Autodesk Inventor part; units mm, degrees
ref_plane "YZ Plane" through (0, 0, 0) normal (1, 0, 0) x (0, 1, 0)
ref_plane "XZ Plane" through (0, 0, 0) normal (0, 1, 0) x (-1, 0, 0)
ref_plane "XY Plane" through (0, 0, 0) normal (0, 0, 1) x (1, 0, 0)
sketch "Sketch1" plane through (0, 0, 0) normal (0, 0, 1) x (1, 0, 0)
  arc A0 (4.0641, 0.1774) -> (4.0641, -0.1774) centre (0, 0) ccw
  arc A1 (5.6501, 0.2467) -> (5.6501, -0.2467) centre (0, 0) ccw
  line L0 (4.0641, -0.1774) -> (5.6501, -0.2467)
  line L1 (4.0641, 0.1774) -> (5.6501, 0.2467)
  dimension "d0" = 8.1359
  dimension "d13" = 5
  dimension "d26" = 1.5875
extrude "Extrusion3" add sketch "Sketch1" along normal blind 11.9062
fillet "Fillet4" radius 0.7937 4 edges at (5.6501, 0.2467, 5.9531) (4.0641, 0.1774, 5.9531) (4.0641, -0.1774, 5.9531) (5.6501, -0.2467, 5.9531)
sketch "Sketch4" plane through (0, 0, 11.9062) normal (0, 0, 1) x (1, 0, 0)
  arc A0 (5.534, 1.1658) -> (5.534, -1.1658) centre (0, 0) ccw
  arc A1 (0, 5.6555) -> (0, -5.6555) centre (0, 0) ccw
  line L0 (0, 5.6555) -> (-10.3791, 5.6555)
  line L1 (-10.3791, 5.6555) -> (-10.3791, -5.6555)
  line L2 (0, -5.6555) -> (-10.3791, -5.6555)
  dimension "d192" = 10.3791
extrude "Extrusion5" add sketch "Sketch4" against normal up to surface (11.9062 mm away)
sketch "Sketch8" plane through (0, 0, 11.9062) normal (0, 0, 1) x (1, 0, 0)
  arc A0 (3.9806, 0.8386) -> (3.9806, -0.8386) centre (0, 0) ccw
  circle A1 centre (0, 4.068) radius 0.3969
  circle A2 centre (0, -4.068) radius 0.3969
  circle A3 centre (-1.5567, 3.7583) radius 0.3969
  circle A4 centre (-1.5567, -3.7583) radius 0.3969
  circle A5 centre (-2.8765, 2.8765) radius 0.3969
  circle A6 centre (-2.8765, -2.8765) radius 0.3969
  circle A7 centre (1.5567, 3.7583) radius 0.3969
  circle A8 centre (1.5567, -3.7583) radius 0.3969
  circle A9 centre (2.8765, 2.8765) radius 0.3969
  circle A10 centre (2.8765, -2.8765) radius 0.3969
  arc A11 (3.9806, 0.8386) -> (3.9806, -0.8386) centre (0, 0) ccw
  circle A12 centre (3.7583, 1.5567) radius 0.3969
  circle A13 centre (3.7583, -1.5567) radius 0.3969
  point P0 (4.7625, 0)
  dimension "d71" = 4.7625
  dimension "d72" = 0.7937
  dimension "d74" = 0.7937
  dimension "d75" = 0.7937
  dimension "d76" = 22.5
  dimension "d77" = 0.7937
  dimension "d78" = 22.5
  dimension "d110" = 0.7937
  dimension "d111" = 0.7937
  dimension "d112" = 22.5
  dimension "d113" = 22.5
  dimension "d158" = 0.7937
  dimension "d159" = 0.7937
  dimension "d160" = 22.5
  dimension "d161" = 22.5
  dimension "d165" = 0.7937
  dimension "d166" = 0.7937
  dimension "d167" = 22.5
  dimension "d168" = 22.5
  dimension "d171" = 22.5
  dimension "d172" = 0.7937
  dimension "d173" = 0.7937
  dimension "d174" = 22.5
  dimension "d191" = 45
sketch "Sketch22" plane through (-10.3791, -5.6555, 11.9062) normal (-1, 0, 0) x (0, 0, 1)
  line L0 (-4.9752, 8.0367) -> (-3.6004, 5.6555)
  line L1 (-3.6004, 5.6555) -> (-4.9752, 3.2742)
  line L2 (-4.9752, 3.2742) -> (-7.7248, 3.2742)
  line L3 (-7.7248, 3.2742) -> (-9.0996, 5.6555)
  line L4 (-9.0996, 5.6555) -> (-7.7248, 8.0367)
  line L5 (-7.7248, 8.0367) -> (-4.9752, 8.0367)
  line L6 (0, 11.3109) -> (-11.9062, 11.3109)
  line L7 (0, 11.3109) -> (0, 0)
  point P0 (-11.9062, 5.6555)
  point P1 (-6.35, 5.6555)
  dimension "d145" = 4.7625
  dimension "d146" = 5.6555
  dimension "d147" = 6.35
extrude "Extrusion28" cut sketch "Sketch22" against normal up to surface
extrude "Extrusion36" add sketch "Sketch8" against normal up to surface (11.9062 mm away)
ref_plane "Work Plane3" through (-7.2041, -5.6555, 11.9062) normal (-1, 0, 0) x (0, 0, 1)
sketch "Sketch28" plane through (-7.2041, -5.6555, 11.9062) normal (-1, 0, 0) x (0, 0, 1)
  line L0 (-4.9752, 8.0367) -> (-3.6004, 5.6555)
  line L1 (-3.6004, 5.6555) -> (-4.9752, 3.2742)
  line L2 (-4.9752, 3.2742) -> (-7.7248, 3.2742)
  line L3 (-7.7248, 3.2742) -> (-9.0996, 5.6555)
  line L4 (-9.0996, 5.6555) -> (-7.7248, 8.0367)
  line L5 (-7.7248, 8.0367) -> (-4.9752, 8.0367)
  line L6 (-7.7248, 8.0367) -> (-4.9752, 8.0367)
  line L7 (-9.0996, 5.6555) -> (-7.7248, 8.0367)
  line L8 (-3.6004, 5.6555) -> (-4.9752, 3.2742)
  circle A0 centre (-6.35, 5.6555) radius 1.5875
  point P0 (-11.9062, 5.6555)
  dimension "d194" = 3.175
extrude "Extrusion37" add sketch "Sketch28" against normal blind 1.5875
sketch "Sketch29" plane through (-7.2041, -5.6555, 11.9062) normal (-1, 0, 0) x (0, 0, 1)
  circle A0 centre (-6.35, 5.6555) radius 1.5875
  circle A1 centre (-6.35, 5.6555) radius 0.7937
  point P0 (-11.9062, 5.6555)
  dimension "d197" = 1.5875
extrude "Extrusion38" cut sketch "Sketch29" against normal through all contours A1
equation "\"d72\" = d75"
equation "\"d74\" = d75"
equation "\"d77\" = d75"
equation "\"d110\" = d75"
equation "\"d111\" = d75"
equation "\"d158\" = d75"
equation "\"d159\" = d75"
equation "\"d165\" = d75"
equation "\"d166\" = d75"
properties part number "claww"
Verification items for the finished model (mm, model axes). A direction names the side the tool comes from. Give positions to 0.01 mm unless a question says otherwise; leave off trailing zeros. Loops run counter-clockwise (first coordinate to the right, second up) from the corner with the lowest first, then second, coordinate; pieces in that order, holes last.
1. Section check B-B, the plane x = -7. Enter the section's corners in (y, z) (1 decimal).
2. Go/stop test with flat-tipped pins: pin 1 Ø2.5 at (y, z) = (0.5, 6) entering from -X; pin 2 Ø1 at (x, z) = (2, 10.5) entering from -Y. Record where each tip stops, or that it passes through.
3. Set-up check for faces 1 (the cylindrical face through (4.747, -0.794, 5.542)), 2 (the flat face through (-4.7, -1.2, 3.5)), 3 (the flat face through (-9, 2.381, 6)): record each of +Z, -Z, +X, -X, +Y, -Y from which the full face is reachable in a straight line by a thin tool's end or side.
4. Section check A-A, the plane x = -3.75. Enter the section's corners in (y, z), then the cut area to 3 significant figures.
5. Mould release check, pull along Y, two halves, no side actions. Record for faces 4 (the flat face through (-10.379, 3, 6)), 5 (the cylindrical face through (4, 4, 6)), 6 (the cylindrical face through (-6.42, 0.48, 7.07)): released by +Y, released by -Y, zero draft, split by the parting line, or undercut.
6. Section check C-C, the plane y = 4.5. Enter the section's corners in (x, z), then the cut area to 3 significant figures.
7. Thickness scan on line 1 (X direction, y = -3.5, z = 7.75); line 2 (Y direction, x = 2, z = 9); line 3 (X direction, y = -2.75, z = 0.75). Record the ranges inside material, lowest first.
Geometry says:
1. outline: (-5.7, 0) - (5.7, 0) - (5.7, 11.9) - (-5.7, 11.9) - close; hole circle Ø3.2 at (0, 5.6)
2. pin 1: stops at x = -7.2
2. pin 2: stops at y = -5.45
3. face 1: +X, -X
3. face 2: none
3. face 3: -X
4. outline: (-5.66, 0) - (-1.58, 0) - (-1.58, 3.72) - (-2.38, 4.18) - (-2.38, 6.93) - (-1.58, 7.4) - (-1.58, 11.91) - (-5.66, 11.91) - close; (1.58, 0) - (5.66, 0) - (5.66, 11.91) - (1.58, 11.91) - (1.58, 7.4) - (2.38, 6.93) - (2.38, 4.18) - (1.58, 3.72) - close
4. area: 92.0 mm2
5. face 4: zero draft
5. face 5: released by +Y
5. face 6: undercut
6. outline: (-10.38, 0) - (3.43, 0) - (3.43, 11.91) - (-10.38, 11.91) - close
6. area: 164 mm2
7. line 1: x = -10.38 to -2.07, -1.86 to -1.26, 1.26 to 1.86, 2.07 to 4.44
7. line 2: y = -5.29 to -3.54, 3.54 to 5.29
7. line 3: x = -10.38 to -2.5, 2.5 to 4.94
